Design review of the part built by this model. Coordinates are the model's own, in mm. A direction names the side the tool comes from. Coordinates: 2 decimals unless noted, no trailing zeros. Write each loop counter-clockwise with the first axis right and the second up, starting at its lowest first coordinate (ties: lowest second). Pieces come first, ordered by that corner, then holes. Notation, with made-up numbers: (45, 62.5) -> (91, 62.5) arc R35 ccw to (91, 100.5) -> close; hole circle Ø8 at (61, 31.25). An arc over 180 degrees is marked (long way). One line per question, with ' | ' between items. Start each with the question number.
Q1. For faces 1 (the flat face through (6.5, 0, 0.2)), 2 (the flat face through (11, -80, -11)), list the 3-axis set-ups (+Z, -Z, +X, -X, +Y, -Y) from which the entire face can be reached by the end or side of a thin tool; tool diameter is ignored.
Q2. Add section B-B on z = 0. State the section outline as (x, y) points, and give its area (3 significant figures).
Q3. Draft analysis for pull direction Z (two halves, no side actions). For faces 3 (the cylindrical face through (-14.985, -74.93, 0.66)), 4 (the flat face through (-1.7, 20, -22.1)), 5 (the flat face through (6.5, -70, 0.2)), state which applies: pulls with the +Z half, pulls with the -Z half, needs draft (parallel to the pull), parting line crosses it, or undercut.
Q4. Add section A-A on x = 0. State the section outline as (y, z) points.
Q5. Wall thickness on probe 1 along Z at (x, y) = (0, -29.5); probe 2 along Z at (x, y) = (0, 3.25); probe 3 along Y at (x, z) = (-7.5, 6): over which ranges is each line inside the solid? List them lowest first.
Q6. Add section C-C on y = -8.5. State the section outline as (x, z) points.
Q7. For P1, Ø5, axis at x = 10.5, z = 4, coming from the +Y side; P2, Ø19, axis at x = 0, z = 0, coming from the -Y side; P3, Ø8, axis at x = -15, y = -68.5, coming from the -Z side, all flat-tipped, find the tip position at first contact; note any pin that passes through.
from build123d import *

# Parameters (mm, degrees)
F0_R     = 25
F0_R_2   = 6
F1_DEPTH = 70
F2_R     = 25
F2_R_2   = 15
F3_DEPTH = 10
F4_R     = 25
F4_R_2   = 15
F5_DEPTH = 20
F6_SIZE  = 7


with BuildPart() as f1:
    # F0 (on Front) → F1 (new body)
    with BuildSketch(Plane.XZ):
        Circle(F0_R)
        Circle(F0_R_2, mode=Mode.SUBTRACT)
    extrude(amount=F1_DEPTH)

    # F2 (on face) → F3 (join)
    with BuildSketch(Plane.XZ.offset(70)):
        Circle(F2_R)
        Circle(F2_R_2, mode=Mode.SUBTRACT)
    extrude(amount=F3_DEPTH)

    # F4 (on face) → F5 (join)
    with BuildSketch(Plane(origin=(0, 0, 0), x_dir=(-1, 0, 0), z_dir=(0, 1, 0))):
        Circle(F4_R)
        Circle(F4_R_2, mode=Mode.SUBTRACT)
    extrude(amount=F5_DEPTH)

    # F6
    f6_edges = [f1.edges().sort_by_distance(p)[0] for p in [
        (15, 20, 0),
    ]]
    chamfer(f6_edges, length=F6_SIZE)


solid = f1.part
Output values:
1) face 1: +Y | face 2: +Z, -Z, +X, -X, -Y
2) outline: (-25, -80) -> (-15, -80) -> (-15, -70) -> (-6, -70) -> (-6, 0) -> (-15, 0) -> (-15, 13) -> (-22, 20) -> (-25, 20) -> close; (6, -70) -> (15, -70) -> (15, -80) -> (25, -80) -> (25, 20) -> (22, 20) -> (15, 13) -> (15, 0) -> (6, 0) -> close | area: 3,210 mm2
3) face 3: undercut | face 4: needs draft | face 5: undercut
4) outline: (-80, -25) -> (20, -25) -> (20, -22) -> (13, -15) -> (0, -15) -> (0, -6) -> (-70, -6) -> (-70, -15) -> (-80, -15) -> close; (-80, 15) -> (-70, 15) -> (-70, 6) -> (0, 6) -> (0, 15) -> (13, 15) -> (20, 22) -> (20, 25) -> (-80, 25) -> close
5) probe 1: z = -25 to -6, 6 to 25 | probe 2: z = -25 to -15, 15 to 25 | probe 3: y = -70 to 0
6) outline: circle Ø50 at (0, 0); hole circle Ø12 at (0, 0)
7) P1: stops at y = 0 | P2: stops at y = -70 | P3: stops at z = -22.45
